```python
from build123d import *

# Parameters (mm, degrees)
SKETCH1_W               = 15.377554838
SKETCH1_H               = 42.931213808
SKETCH1_R               = 3.129225598
BOSS_EXTRUDE1_DEPTH     = 15
CUT_EXTRUDE1_DEPTH      = 1
CUT_EXTRUDE1_DEPTH_BACK = 16.377554838


with BuildPart() as part:
    # Sketch1 → Boss-Extrude1 (new body)
    with BuildSketch(Plane.XY):
        with Locations((215.9, 0)):
            Rectangle(SKETCH1_W, SKETCH1_H)
        with Locations((215.9, -12.7)):
            Circle(SKETCH1_R, mode=Mode.SUBTRACT)
        with Locations((215.9, 12.7)):
            Circle(SKETCH1_R, mode=Mode.SUBTRACT)
    extrude(amount=BOSS_EXTRUDE1_DEPTH)

    # Sketch2 → Cut-Extrude1 (cut, two sides)
    with BuildSketch(Plane(origin=(223.588777419, 0, 0), x_dir=(0, 0, -1), z_dir=(1, 0, 0))) as cut_extrude1_sk:
        with BuildLine():
            Line((0, -3.075), (-3.075, -3.075))
            ThreePointArc((-3.075, -3.075), (-6.15, 0), (-3.075, 3.075))
            Line((-3.075, 3.075), (0, 3.075))
            ThreePointArc((0, 3.075), (3.075, 0), (0, -3.075))
        make_face()
    extrude(amount=CUT_EXTRUDE1_DEPTH, mode=Mode.SUBTRACT)
    extrude(cut_extrude1_sk.sketch, amount=-CUT_EXTRUDE1_DEPTH_BACK, mode=Mode.SUBTRACT)


solid = part.part
```
Check sheet for the modelled part. Datum: model origin and axes. Units: mm. A direction names the side the tool comes from. Give positions to 0.01 mm unless a question says otherwise; leave off trailing zeros. Write each loop counter-clockwise with the first axis right and the second up, starting at its lowest first coordinate (ties: lowest second). Pieces come first, ordered by that corner, then holes.
Item 1: Gauge pin test, flat end, axial feed: pin 1 (1 mm diameter, centred on x = 218.5, y = -1.5, fed in from -Z). Record the tip position at first contact, or that the pin passes through.
Item 2: Cross-section at A-A (x = 215.9). Enter the section's corners in (y, z) (3 decimals), and give its area (3 significant figures).
Item 3: Scan lines: L1, parallel to Y at x = 215.9, z = 10.75; L2, parallel to Y at x = 215.75, z = 1.5 (3 decimals); L3, parallel to Y at x = 215.9, z = 5.5. Record each from-to range of solid material in increasing order.
Item 4: Cross-section at B-B (y = 12.7). Enter the section's corners in (x, z), and give its area (3 significant figures).
Item 5: Draft check along Y on faces 1 (the face through (216.01, -0.07, 6.15)), 2 (the face through (216, 21.466, 7)), 3 (the face through (216, -21.466, 7)). Enter one of: released by +Y, released by -Y, zero draft, split by the parting line, or undercut.
Item 6: Access from +Z, -Z, +X, -X, +Y, -Y to the whole of each face (thin tool, end or side, straight path). Record for faces 4 (the face through (216, -3.075, 2)), 5 (the face through (208.211, 0, 7)).
Item 7: Cross-section at D-D (x = 222.25). Enter the section's corners in (y, z) (3 decimals), and give its area (3 significant figures).
Item 8: Cross-section at C-C (z = 4.75). Enter the section's corners in (x, y), and give its area (3 significant figures).
Report:
1. pin 1: stops at z = 5.41
2. outline: (-21.466, 0) - (-15.829, 0) - (-15.829, 15) - (-21.466, 15) - close; (-9.571, 0) - (-3.075, 0) - (-3.075, 3.075) arc R3.075 cw to (3.075, 3.075) - (3.075, 0) - (9.571, 0) - (9.571, 15) - (-9.571, 15) - close; (15.829, 0) - (21.466, 0) - (21.466, 15) - (15.829, 15) - close
2. area: 422 mm2
3. L1: y = -21.47 to -15.83, -9.57 to 9.57, 15.83 to 21.47
3. L2: y = -21.466 to -15.826, -9.574 to -3.075, 3.075 to 9.574, 15.826 to 21.466
3. L3: y = -21.47 to -15.83, -9.57 to -1.89, 1.89 to 9.57, 15.83 to 21.47
4. outline: (208.21, 0) - (212.77, 0) - (212.77, 15) - (208.21, 15) - close; (219.03, 0) - (223.59, 0) - (223.59, 15) - (219.03, 15) - close
4. area: 137 mm2
5. face 1: undercut
5. face 2: released by +Y
5. face 3: released by -Y
6. face 4: -Z, +X, -X
6. face 5: +Z, -Z, -X, +Y, -Y
7. outline: (-21.466, 0) - (-3.075, 0) - (-3.075, 3.075) arc R3.075 cw to (3.075, 3.075) - (3.075, 0) - (21.466, 0) - (21.466, 15) - (-21.466, 15) - close
7. area: 610 mm2
8. outline: (208.21, -21.47) - (223.59, -21.47) - (223.59, -2.58) - (208.21, -2.58) - close; (208.21, 2.58) - (223.59, 2.58) - (223.59, 21.47) - (208.21, 21.47) - close; hole circle Ø6.26 at (215.9, -12.7); hole circle Ø6.26 at (215.9, 12.7)
8. area: 519 mm2
